from build123d import *

# Parameters (mm, degrees)
SKETCH1_R           = 1.720095417
SKETCH1_R_2         = 1.632335783
SKETCH1_R_3         = 3.048
BOSS_EXTRUDE1_DEPTH = 6.35


with BuildPart() as part:
    # Sketch1 → Boss-Extrude1 (new body)
    with BuildSketch(Plane.XY):
        with BuildLine():
            Line((0.359622665, 84.647626996), (0.359622665, 112.547896558))
            ThreePointArc((0.359622665, 112.547896558), (1.569792033, 115.17822767), (4.285435965, 116.18243367))
            Line((4.285435965, 116.18243367), (699.960441306, 116.18243367))
            Line((699.960441306, 116.18243367), (699.960441306, 131.904163347))
            ThreePointArc((699.960441306, 131.904163347), (701.183091811, 134.700225562), (704.024750828, 135.812795653))
            Line((704.024750828, 135.812795653), (867.944172073, 135.812795653))
            Line((867.944172073, 135.812795653), (867.944172073, 130.611938178))
            Line((867.944172073, 130.611938178), (867.944172073, 124.543323228))
            Line((867.944172073, 124.543323228), (714.00720644, 124.543323228))
            Line((714.00720644, 124.543323228), (714.00720644, 104.995667719))
            Line((714.00720644, 104.995667719), (12.71320644, 104.995667719))
            Line((12.71320644, 104.995667719), (12.71320644, 91.663924817))
            Line((12.71320644, 91.663924817), (714.00720644, 91.663924817))
            Line((714.00720644, 91.663924817), (714.00720644, 72.51225313))
            Line((714.00720644, 72.51225313), (935.984655082, 72.51225313))
            Line((935.984655082, 72.51225313), (935.984655082, 124.543323228))
            Line((935.984655082, 124.543323228), (933.071984653, 124.543323228))
            Line((933.071984653, 124.543323228), (933.071984653, 135.812795653))
            Line((933.071984653, 135.812795653), (946.192785632, 135.812795653))
            ThreePointArc((946.192785632, 135.812795653), (948.657072186, 134.878542119), (949.738968911, 132.475411377))
            Line((949.738968911, 132.475411377), (949.738968911, 115.492795653))
            Line((949.738968911, 115.492795653), (1145.318968911, 115.492795653))
            ThreePointArc((1145.318968911, 115.492795653), (1147.47423038, 114.600057122), (1148.366968911, 112.444795653))
            Line((1148.366968911, 112.444795653), (1148.366968911, 83.61670663))
            ThreePointArc((1148.366968911, 83.61670663), (1147.47423038, 81.461445161), (1145.318968911, 80.56870663))
            Line((1145.318968911, 80.56870663), (949.738968911, 80.56870663))
            Line((949.738968911, 80.56870663), (949.738968911, 64.012598058))
            ThreePointArc((949.738968911, 64.012598058), (948.74540471, 61.39621374), (946.192785632, 60.24870663))
            Line((946.192785632, 60.24870663), (704.024750828, 60.24870663))
            ThreePointArc((704.024750828, 60.24870663), (701.213068629, 61.288906282), (699.960441306, 64.012598058))
            Line((699.960441306, 64.012598058), (699.960441306, 81.011908201))
            Line((699.960441306, 81.011908201), (4.285435965, 81.011908201))
            ThreePointArc((4.285435965, 81.011908201), (1.569547298, 82.016705042), (0.359622665, 84.647626996))
        make_face()
        with Locations((94.1622142, 88.091107164)):
            Circle(SKETCH1_R, mode=Mode.SUBTRACT)
        with Locations((94.1622142, 108.484732819)):
            Circle(SKETCH1_R, mode=Mode.SUBTRACT)
        with Locations((221.392126764, 108.484732819)):
            Circle(SKETCH1_R, mode=Mode.SUBTRACT)
        with Locations((221.392126764, 88.091107164)):
            Circle(SKETCH1_R, mode=Mode.SUBTRACT)
        with Locations((348.078760153, 108.484732819)):
            Circle(SKETCH1_R, mode=Mode.SUBTRACT)
        with Locations((348.078760153, 88.091107164)):
            Circle(SKETCH1_R_2, mode=Mode.SUBTRACT)
        with Locations((475.146430575, 108.484732819)):
            Circle(SKETCH1_R, mode=Mode.SUBTRACT)
        with Locations((475.146430575, 88.091107164)):
            Circle(SKETCH1_R, mode=Mode.SUBTRACT)
        with Locations((602.130384222, 88.091107164)):
            Circle(SKETCH1_R, mode=Mode.SUBTRACT)
        with Locations((602.130384222, 108.484732819)):
            Circle(SKETCH1_R, mode=Mode.SUBTRACT)
        with Locations((705.892847696, 116.18243367)):
            Circle(SKETCH1_R, mode=Mode.SUBTRACT)
        with Locations((705.892847696, 81.011908201)):
            Circle(SKETCH1_R, mode=Mode.SUBTRACT)
        with Locations((760.070975046, 130.611938178)):
            Circle(SKETCH1_R, mode=Mode.SUBTRACT)
        with Locations((760.070975046, 66.505299661)):
            Circle(SKETCH1_R, mode=Mode.SUBTRACT)
        with Locations((848.138968911, 130.611938178)):
            Circle(SKETCH1_R, mode=Mode.SUBTRACT)
        with Locations((848.138968911, 66.505299661)):
            Circle(SKETCH1_R, mode=Mode.SUBTRACT)
        with Locations((943.890172073, 116.18243367)):
            Circle(SKETCH1_R, mode=Mode.SUBTRACT)
        with Locations((943.890172073, 81.011908201)):
            Circle(SKETCH1_R, mode=Mode.SUBTRACT)
        with Locations((1023.106655082, 98.527788179)):
            Circle(SKETCH1_R_3, mode=Mode.SUBTRACT)
        with Locations((1099.420523291, 98.527788179)):
            Circle(SKETCH1_R_3, mode=Mode.SUBTRACT)
    extrude(amount=BOSS_EXTRUDE1_DEPTH)


solid = part.part
Build history of the part. All positions in model axes, mm. Round coordinates to 2 decimals unless told otherwise and drop trailing zeros. Write each loop counter-clockwise with the first axis right and the second up, starting at its lowest first coordinate (ties: lowest second). Pieces come first, ordered by that corner, then holes. Notation, with made-up numbers: M 2,65.25 L 60,65.25 A20 cw 60,102.25 Z; hole C 72,4 d8. An arc over 180 degrees is marked long. Answer as a JSON object with one key per item and string values. Group by question number.
(1) Cut at C-C (x = 1055). Give the cut face in (y, z).
(2) Cut at A-A (x = 108). Give the cut face in (y, z), and give its area (3 significant figures).
(3) Flat gauge pins, fed straight in: pin 1 (3 mm diameter, centred on y = 127.5, z = 4, fed in from +X); pin 2 (1.9 mm diameter, centred on x = 885, z = 1.5, fed in from -Y); pin 3 (3 mm diameter, centred on x = 368.5, z = 4, fed in from -Y). Where does each tip first touch, or does it go through?
(4) Cut at B-B (z = 2). Give the number of separate pieces and of enclosed holes in the cut face, and give its area (3 significant figures).
(5) Drill centre lines: L1, parallel to X at y = 67, z = 0.75; L2, parallel to Y at x = 340.5, z = 1; L3, parallel to Y at x = 603, z = 2.75. Where is each one in solid material? Low to high.
Responses:
{
 "1": {"outline": "M 80.57,0 L 115.49,0 L 115.49,6.35 L 80.57,6.35 Z"},
 "2": {"outline": "M 81.01,0 L 91.66,0 L 91.66,6.35 L 81.01,6.35 Z; M 105,0 L 116.18,0 L 116.18,6.35 L 105,6.35 Z", "area": "139 mm2"},
 "3": {"pin 1": "stops at x = 949.74", "pin 2": "stops at y = 60.25", "pin 3": "stops at y = 81.01"},
 "4": {"separate pieces": "1", "enclosed holes": "20", "area": "28,500 mm2"},
 "5": {"L1": "x = 699.96 to 758.42, 761.72 to 846.49, 849.79 to 949.74", "L2": "y = 81.01 to 91.66, 105 to 116.18", "L3": "y = 81.01 to 86.61, 89.58 to 91.66, 105 to 107, 109.97 to 116.18"}
}
